Part model, mm, in its own coordinate system. Round coordinates to 2 decimals unless told otherwise and drop trailing zeros. Loops run counter-clockwise (first coordinate to the right, second up) from the corner with the lowest first, then second, coordinate; pieces in that order, holes last.
(1) Probe probe 1 along Y at (x, z) = (-100, 3.7); probe 2 along X at (y, z) = (0.5, 1.9); probe 3 along X at (y, z) = (-1.5, 1.85). List the from-to ranges inside material, lowest first.
(2) Mould opens along Y. For faces 1 (the face through (-107, 0, 2)), 2 (the face through (-51, -3, 5)), 3 (the face through (-98.092, 0.601, 2.465)) say: +Y half, -Y half, draft (parallel to the pull), parting line (faces both ways), or undercut.
(3) Cut at A-A on x = -50. List the corners of the cut face in (y, z).
(4) Cut at B-B on y = 0. List the corners of the cut face in (x, z).
(5) Cut at D-D on y = -4.25. List the corners of the cut face in (x, z).
(6) Flat gauge pins, fed straight in: pin 1 (4.5 mm diameter, centred on x = 0, y = 0, fed in from -Z); pin 2 (2 mm diameter, centred on y = 2, z = 2, fed in from +X). Where does each tip first touch, or does it go through?
(7) Cut at C-C on z = 2.95. List the corners of the cut face in (x, y).
from build123d import *

# Parameters (mm, degrees)
F0_R     = 2
F1_DEPTH = 5


with BuildPart() as f1:
    # F0 (on Top) → F1 (new body)
    with BuildSketch(Plane.XY):
        with BuildLine():
            ThreePointArc((0, -7), (7, 0), (0, 7))
            Line((0, 7), (-100, 7))
            ThreePointArc((-100, 7), (-107, 0), (-100, -7))
            Line((-100, -7), (0, -7))
        make_face()
        with Locations((-100, 0)):
            Circle(F0_R, mode=Mode.SUBTRACT)
        with Locations((-50, 0)):
            Circle(F0_R, mode=Mode.SUBTRACT)
        Circle(F0_R, mode=Mode.SUBTRACT)
    extrude(amount=F1_DEPTH)


solid = f1.part
Final values:
1. probe 1: y = -7 to -2, 2 to 7
1. probe 2: x = -106.98 to -101.94, -98.06 to -51.94, -48.06 to -1.94, 1.94 to 6.98
1. probe 3: x = -106.84 to -101.32, -98.68 to -51.32, -48.68 to -1.32, 1.32 to 6.84
2. face 1: parting line
2. face 2: draft
2. face 3: undercut
3. outline: (-7, 0) - (-2, 0) - (-2, 5) - (-7, 5) - close; (2, 0) - (7, 0) - (7, 5) - (2, 5) - close
4. outline: (-107, 0) - (-102, 0) - (-102, 5) - (-107, 5) - close; (-98, 0) - (-52, 0) - (-52, 5) - (-98, 5) - close; (-48, 0) - (-2, 0) - (-2, 5) - (-48, 5) - close; (2, 0) - (7, 0) - (7, 5) - (2, 5) - close
5. outline: (-105.56, 0) - (5.56, 0) - (5.56, 5) - (-105.56, 5) - close
6. pin 1: stops at z = 0
6. pin 2: stops at x = 6.93
7. outline: (-100, -7) - (0, -7) arc R7 ccw to (0, 7) - (-100, 7) arc R7 ccw to start; hole circle Ø4 at (-100, 0); hole circle Ø4 at (-50, 0); hole circle Ø4 at (0, 0)
